Can you work these out from the model? Positions are in its coordinate system, mm. Face numbers are marked on the shaded views. A direction names the side the tool comes from. Coordinates: 2 decimals unless noted, no trailing zeros. Write each loop counter-clockwise with the first axis right and the second up, starting at its lowest first coordinate (ties: lowest second). Pieces come first, ordered by that corner, then holes. Notation, with made-up numbers: M 6.5,19.25 L 37.5,19.25 A17 ccw 37.5,37.25 Z; hole C 36.5,21.25 d10. An arc over 180 degrees is marked long. Answer as a JSON object with one key per item and string values. Group by question number.
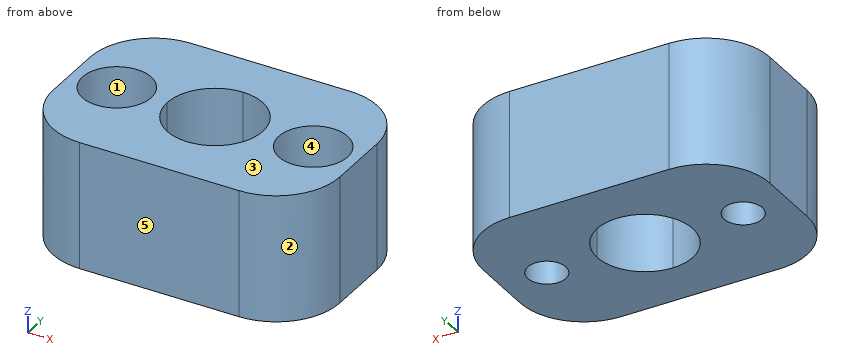
from build123d import *

# Parameters (mm, degrees)
BOSS_EXTRUDE1_DEPTH = 12.7
FILLET1_R           = 6.35
SKETCH2_R           = 3.429
CUT_EXTRUDE1_DEPTH  = 6.35


with BuildPart() as part:
    # Sketch1 → Boss-Extrude1 (new body)
    with BuildSketch(Plane.XY):
        with BuildLine():
            Line((-14.2875, -4.7625), (-14.2875, 0))
            Line((-14.2875, 0), (-28.575, 0))
            Line((-28.575, 0), (-28.575, -9.525))
            Line((-28.575, -9.525), (-25.9715, -9.525))
            ThreePointArc((-25.9715, -9.525), (-24.0665, -7.62), (-22.1615, -9.525))
            Line((-22.1615, -9.525), (-19.05, -9.525))
            ThreePointArc((-19.05, -9.525), (-17.655096045, -6.157403955), (-14.2875, -4.7625))
        make_face()
        with BuildLine():
            ThreePointArc((-14.2875, -14.2875), (-17.655096045, -12.892596045), (-19.05, -9.525))
            Line((-19.05, -9.525), (-22.1615, -9.525))
            ThreePointArc((-22.1615, -9.525), (-24.0665, -11.43), (-25.9715, -9.525))
            Line((-25.9715, -9.525), (-28.575, -9.525))
            Line((-28.575, -9.525), (-28.575, -19.05))
            Line((-28.575, -19.05), (-14.2875, -19.05))
            Line((-14.2875, -19.05), (-14.2875, -14.2875))
        make_face()
        with BuildLine():
            Line((-6.4135, -9.525), (-9.525, -9.525))
            ThreePointArc((-9.525, -9.525), (-10.919903955, -12.892596045), (-14.2875, -14.2875))
            Line((-14.2875, -14.2875), (-14.2875, -19.05))
            Line((-14.2875, -19.05), (0, -19.05))
            Line((0, -19.05), (0, -9.525))
            Line((0, -9.525), (-2.6035, -9.525))
            ThreePointArc((-2.6035, -9.525), (-4.5085, -11.43), (-6.4135, -9.525))
        make_face()
        with BuildLine():
            Line((0, 0), (-14.2875, 0))
            Line((-14.2875, 0), (-14.2875, -4.7625))
            ThreePointArc((-14.2875, -4.7625), (-10.919903955, -6.157403955), (-9.525, -9.525))
            Line((-9.525, -9.525), (-6.4135, -9.525))
            ThreePointArc((-6.4135, -9.525), (-4.5085, -7.62), (-2.6035, -9.525))
            Line((-2.6035, -9.525), (0, -9.525))
            Line((0, -9.525), (0, 0))
        make_face()
    extrude(amount=BOSS_EXTRUDE1_DEPTH)

    # Fillet1
    fillet1_edges = [part.edges().sort_by_distance(p)[0] for p in [
        (-28.575, -19.05, 6.35),
        (-28.575, 0, 6.35),
        (0, 0, 6.35),
        (0, -19.05, 6.35),
    ]]
    fillet(fillet1_edges, radius=FILLET1_R)

    # Sketch2 → Cut-Extrude1 (cut)
    with BuildSketch(Plane.XY.offset(12.7)):
        with Locations((-24.0665, -9.525)):
            Circle(SKETCH2_R)
        with Locations((-4.5085, -9.525)):
            Circle(SKETCH2_R)
    extrude(amount=-CUT_EXTRUDE1_DEPTH, mode=Mode.SUBTRACT)


solid = part.part
Q1. If we section it at B-B on x = -24.5: List the corners of the cut face in (y, z) for me, and give its area (3 significant figures).
Q2. We'd pull the mould along X, two halves only. Please class the marked faces 1, 2 and 3: pulls with the +X half, pulls with the -X half, needs draft (parallel to the pull), parting line crosses it, or undercut.
Q3. If we section it at C-C on y = -5.25: List the corners of the cut face in (x, z) for me.
Q4. On a 3-axis mill with a long thin cutter (end or side, diameter ignored), from which of +Z, -Z, +X, -X, +Y, -Y can I reach the whole of each face in a straight line? I mean the marked faces 4 and 5. Say none if no direction works.
Q5. Please list where these lines run through material, in increasing order: L1, parallel to X at y = -9.75, z = 2.75 (3 decimals); L2, parallel to X at y = -11, z = 8 (3 decimals); L3, parallel to Y at x = -10.75, z = 10.5.
Q6. Will these pins go through, and if not, where does the flat tip stop? pin 1 (4 mm diameter, centred on x = -24.07, y = -9.52, fed in from +Z); pin 2 (6 mm diameter, centred on y = -14, z = 10.5, fed in from +X); pin 3 (3.5 mm diameter, centred on x = -4.51, y = -9.52, fed in from -Z).
Q7. If we section it at A-A on z = 5.25: Give the number of separate pieces and of enclosed holes in the cut face, and give its area (3 significant figures).
Reply:
{
 "1": {"outline": "M -18.63,0 L -11.38,0 L -11.38,6.35 L -12.93,6.35 L -12.93,12.7 L -18.63,12.7 Z; M -7.67,0 L -0.42,0 L -0.42,12.7 L -6.12,12.7 L -6.12,6.35 L -7.67,6.35 Z", "area": "164 mm^2"},
 "2": {"face 1": "undercut", "face 2": "pulls with the +X half", "face 3": "needs draft"},
 "3": {"outline": "M -28.48,0 L -16.39,0 L -16.39,12.7 L -28.48,12.7 Z; M -12.19,0 L -0.1,0 L -0.1,12.7 L -12.19,12.7 Z"},
 "4": {"face 4": "+Z", "face 5": "+Z, -Z, +X, -X, -Y"},
 "5": {"L1": "-28.575 to -25.958, -22.175 to -19.045, -9.53 to -6.4, -2.617 to 0", "L2": "-28.575 to -27.162, -20.971 to -18.816, -9.759 to -7.604, -1.413 to 0", "L3": "-19.05 to -12.71, -6.34 to 0"},
 "6": {"pin 1": "z = 6.35", "pin 2": "x = 0", "pin 3": "through"},
 "7": {"separate pieces": "1", "enclosed holes": "3", "area": "416 mm^2"}
}
